from build123d import *

# Parameters (mm, degrees)
SKETCH_4_W           = 70
SKETCH_4_H           = 35
EXTRUDE_6_DEPTH      = 17.5
EXTRUDE_7_DEPTH      = 5
SHELL_START          = -16.5
SHELL_3_OUTLINE_W    = 69
SHELL_3_OUTLINE_H    = 33
SHELL_3_DEPTH        = 33
SHELL_START_2        = 16.5
SHELL_3_2_DEPTH      = 5
SKETCH_9_W           = 70
SKETCH_9_H           = 4
CUT_EXTRUDE_1_DEPTH  = 6
SKETCH_22_W          = 50
SKETCH_22_H          = 26
EXTRUDE_8_DEPTH      = 13
SHELL_START_3        = -50
SHELL_4_OUTLINE_W    = 24
SHELL_4_OUTLINE_H    = 24
SHELL_4_DEPTH        = 50
SKETCH_23_W          = 24
SKETCH_23_H          = 24
CUT_EXTRUDE_3_DEPTH  = 1
EXTRUDE_11_DEPTH     = 13
SHELL_START_4        = -12
SHELL_13_DEPTH       = 24
CUT_EXTRUDE_16_REACH = 85.741
SKETCH_40_W          = 25
SKETCH_40_H          = 24


# Read off the part's stored shape, not the designer's step: 抽壳3, 抽壳4, 抽壳13
with BuildPart() as part:
    # 草图4 → 凸台-拉伸6 (new, symmetric)
    with BuildSketch(Plane.XY):
        with Locations((35, 0)):
            Rectangle(SKETCH_4_W, SKETCH_4_H)
    extrude(amount=EXTRUDE_6_DEPTH, both=True)

    # 草图6 → 凸台-拉伸7 (add)
    with BuildSketch(Plane.XY.offset(22.5)):
        with BuildLine():
            Line((5, 5), (65, 5))
            ThreePointArc((65, 5), (70, 0), (65, -5))
            Line((65, -5), (5, -5))
            ThreePointArc((5, -5), (0, 0), (5, 5))
        make_face()
    extrude(amount=-EXTRUDE_7_DEPTH)

    # 抽壳3 outline → 抽壳3 (cut)
    with BuildSketch(Plane.XY.offset(SHELL_START)):
        with Locations((35.5, 0)):
            Rectangle(SHELL_3_OUTLINE_W, SHELL_3_OUTLINE_H)
    extrude(amount=SHELL_3_DEPTH, mode=Mode.SUBTRACT)

    # Shell 3 2 outline → Shell 3 2 (cut)
    with BuildSketch(Plane.XY.offset(SHELL_START_2)):
        with BuildLine():
            ThreePointArc((5, 4), (1, 0), (5, -4))
            Line((5, -4), (65, -4))
            ThreePointArc((65, -4), (69, 0), (65, 4))
            Line((65, 4), (5, 4))
        make_face()
    extrude(amount=SHELL_3_2_DEPTH, mode=Mode.SUBTRACT)

    # 草图9 → 切除-拉伸1 (cut)
    with BuildSketch(Plane.XZ.offset(5)):
        with Locations((35, 19.5)):
            Rectangle(SKETCH_9_W, SKETCH_9_H)
    extrude(amount=-CUT_EXTRUDE_1_DEPTH, mode=Mode.SUBTRACT)

    # 草图22 → 凸台-拉伸8 (add, symmetric)
    with BuildSketch(Plane.XY):
        with Locations((-25, 0)):
            Rectangle(SKETCH_22_W, SKETCH_22_H)
    extrude(amount=EXTRUDE_8_DEPTH, both=True)

    # 抽壳4 outline → 抽壳4 (cut)
    with BuildSketch(Plane.YZ.offset(SHELL_START_3)):
        Rectangle(SHELL_4_OUTLINE_W, SHELL_4_OUTLINE_H)
    extrude(amount=SHELL_4_DEPTH, mode=Mode.SUBTRACT)

    # 草图23 → 切除-拉伸3 (cut)
    with BuildSketch(Plane.ZY):
        Rectangle(SKETCH_23_W, SKETCH_23_H)
    extrude(amount=-CUT_EXTRUDE_3_DEPTH, mode=Mode.SUBTRACT)

    # 草图28 → 凸台-拉伸11 (add, symmetric)
    with BuildSketch(Plane(origin=(0, 0, 0), x_dir=(1, 0, 0), z_dir=(0, 1, 0))):
        Polygon((-50, 13), (-50, -13), (-76, -13), align=None)
    extrude(amount=EXTRUDE_11_DEPTH, both=True)

    # 抽壳13 outline → 抽壳13 (cut)
    with BuildSketch(Plane(origin=(0, 0, 0), x_dir=(1, 0, 0), z_dir=(0, 1, 0)).offset(SHELL_START_4)):
        Polygon((-50, 11.585786438), (-73.585786438, -12), (-50, -12), align=None)
    extrude(amount=SHELL_13_DEPTH, mode=Mode.SUBTRACT)

    # 切除-拉伸16: up to this plane
    cut_extrude_16_end = Plane(origin=(-75.646446609, 13, 13.353553391), z_dir=(0.7071067811865512, 0, 0.7071067811865439))
    # 草图40 → 切除-拉伸16 (cut, up to the surface)
    with BuildSketch(Plane.XY.offset(13), mode=Mode.PRIVATE) as cut_extrude_16_sk1:
        with Locations((-62.5, 0)):
            Rectangle(SKETCH_40_W, SKETCH_40_H)
    cut_extrude_16_tool1 = split(extrude(cut_extrude_16_sk1.sketch, amount=-CUT_EXTRUDE_16_REACH, mode=Mode.PRIVATE), bisect_by=cut_extrude_16_end, keep=Keep.BOTH, mode=Mode.PRIVATE)
    add(cut_extrude_16_tool1.solids().sort_by_distance((-62.5, 0, 13))[0], mode=Mode.SUBTRACT)


solid = part.part
Read the model definition and answer for the solid it produces. Units are mm, in the model's axes. A direction names the side the tool comes from. Give positions to 0.01 mm unless a question says otherwise; leave off trailing zeros. Loops run counter-clockwise (first coordinate to the right, second up) from the corner with the lowest first, then second, coordinate; pieces in that order, holes last. Notation, with made-up numbers: (33.25, 28) - (59.25, 28) arc R18 cw to (59.25, 47) - close; hole circle Ø1 at (5.25, 87.5). An arc over 180 degrees is marked (long way). Answer as CSV lines item,"result". Start each with the question number.
1) Find section A-A (y = 7.5). Write down the section's boundary in (x, z), then the cut area to 3 significant figures.
2) Determine the mould class of faces 6 (the face through (-63, 0, 0)), 7 (the face through (-29, -12, 0)), 8 (the face through (35, 17.5, 0)), 9 (the face through (-29, 12, 0)) for opening direction Y: released by +Y, released by -Y, zero draft, split by the parting line, or undercut.
3) Each of these flat-tipped pins is pushed along its axis until it touches: pin 1 Ø13 at (x, y) = (-39.5, 4.5) entering from +Z; pin 2 Ø0.8 at (x, z) = (0.5, 20) entering from -Y; pin 3 Ø20 at (x, z) = (-54, 3.5) entering from -Y. Where does it stop, or does it pass through?
4) Straight lines are drawn through the part: L1, parallel to Y at x = 54, z = 4; L2, parallel to Z at x = -18, y = 5.5. For each, find the intervals that lie inside material, in ascending order. Write a range as from..to.
5) Which of the six approach directions +Z, -Z, +X, -X, +Y, -Y give full straight-line access (tool end or side, diameter ignored) to faces 1 (the face through (-25, 0, -13)), 2 (the face through (-30, 13, 0)), 3 (the face through (-25, 0, -12)), 4 (the face through (-30, 0, 13)), 5 (the face through (1.993, 2.638, 18.409))?
6) Find section D-D (x = 43). Write down the section's boundary in (y, z), then the cut area to 3 significant figures.
7) Find section B-B (x = -21.5). Write down the section's boundary in (y, z), then the cut area to 3 significant figures.
8) Find section C-C (z = 15). Write down the section's boundary in (x, y).
Findings below:
1,outline,"(-76, 13) - (-50, -13) - (0, -13) - (0, -17.5) - (70, -17.5) - (70, -16.5) - (1, -16.5) - (1, -12) - (-50, -12) - (-50, -12.29) - (-75, 12.71) - (-75, 13) - close; (-50, 12) - (1, 12) - (1, 16.5) - (70, 16.5) - (70, 17.5) - (0, 17.5) - (0, 13) - (-50, 13) - close"
1,area,"267 mm^2"
2,face 6,"zero draft"
2,face 7,"undercut"
2,face 8,"released by +Y"
2,face 9,"undercut"
3,pin 1,"z = 13"
3,pin 2,"y = 1"
3,pin 3,"y = -13"
4,L1,"-17.5..-16.5, 16.5..17.5"
4,L2,"-13..-12, 12..13"
5,face 1,"-Z, -X, +Y, -Y"
5,face 2,"+Z, -Z, -X, +Y"
5,face 3,"+X"
5,face 4,"+Z, -X, +Y, -Y"
5,face 5,"none"
6,outline,"(-17.5, -17.5) - (17.5, -17.5) - (17.5, 17.5) - (5, 17.5) - (5, 22.5) - (-5, 22.5) - (-5, 21.5) - (4, 21.5) - (4, 16.5) - (16.5, 16.5) - (16.5, -16.5) - (-16.5, -16.5) - (-16.5, 16.5) - (-4, 16.5) - (-4, 17.5) - (-17.5, 17.5) - close"
6,area,"142 mm^2"
7,outline,"(-13, -13) - (13, -13) - (13, 13) - (-13, 13) - close; hole (-12, -12) - (12, -12) - (12, 12) - (-12, 12) - close"
7,area,"100 mm^2"
8,outline,"(0, -17.5) - (70, -17.5) - (70, -16.5) - (1, -16.5) - (1, 16.5) - (70, 16.5) - (70, 17.5) - (0, 17.5) - close"
